Work out the finished part from the listing and answer in its coordinate system (mm). A direction names the side the tool comes from. Round coordinates to 2 decimals unless told otherwise and drop trailing zeros. Order: outer loops, then holes, each group sorted by start corner. A loop starts at its lowest first (then second) coordinate and runs counter-clockwise, first axis right, second up. Notation, with made-up numbers: (64, 85.25) - (109, 85.25) arc R22 ccw to (109, 120.25) - close; hole circle Ø6 at (74.25, 4). An arc over 180 degrees is marked (long way). Use CSV: the item, a comma, the result in double quotes.
from build123d import *

# Parameters (mm, degrees)
BOSS_EXTRUDE1_DEPTH          = 350
F_3_0_3_DIAMETER_SLOT1_D     = 3
F_3_0_3_DIAMETER_HOLE2_D     = 3
F_3_0_3_DIAMETER_HOLE2_DEPTH = 4


with BuildPart() as part:
    # Sketch1 → Boss-Extrude1 (new body)
    with BuildSketch(Plane(origin=(0, 0, 0), x_dir=(1, 0, 0), z_dir=(0, 1, 0))):
        Polygon((0, 0), (0, 10), (2, 10), (2, 2), (20, 2), (20, 0), align=None)
    extrude(amount=BOSS_EXTRUDE1_DEPTH)

    # Ø3.0 (3) Diameter Slot1 (through all)
    with Locations(Plane.XY):
        with Locations((14.838501141, 25.910104069), (14.838501141, 323.866264903)):
            Hole(F_3_0_3_DIAMETER_SLOT1_D / 2)

    # Ø3.0 (3) Diameter Hole2
    with Locations(Plane(origin=(0, 128.861996081, -176.67995168), x_dir=(0, 1, 0), z_dir=(-1, 0, 0))):
        with Locations((-122.861996081, -170.67995168), (-108.861996081, -170.67995168), (215.138003919, -170.67995168), (201.138003919, -170.67995168)):
            Hole(F_3_0_3_DIAMETER_HOLE2_D / 2, depth=F_3_0_3_DIAMETER_HOLE2_DEPTH)


solid = part.part
(1) For faces 1 (the flat face through (2, 173, -6)), 2 (the flat face through (10, 173, 0)), determine the directions among +Z, -Z, +X, -X, +Y, -Y from which every point of the face is accessible in a straight line to the end or side of a thin tool.
Findings below:
face 1,"-Z, +X, +Y, -Y"
face 2,"+Z, +X, -X, +Y, -Y"
(2) Find the intervals of material crossed by L1, parallel to Z at x = 0.8, y = 20; L2, parallel to Y at x = 1.15, z = -6; L3, parallel to X at y = 302, z = -6.75, in increasing order. Write a range as from..to.
Findings below:
L1,"z = -10..-7.5, -4.5..0"
L2,"y = 0..4.5, 7.5..18.5, 21.5..328.5, 331.5..342.5, 345.5..350"
L3,"x = 0..2"
(3) Find section A-A (z = -6). Determine the outline of the cut face in (x, y), and give its area (3 significant figures).
Findings below:
outline,"(0, 0) - (2, 0) - (2, 4.5) - (0, 4.5) - close; (0, 7.5) - (2, 7.5) - (2, 18.5) - (0, 18.5) - close; (0, 21.5) - (2, 21.5) - (2, 328.5) - (0, 328.5) - close; (0, 331.5) - (2, 331.5) - (2, 342.5) - (0, 342.5) - close; (0, 345.5) - (2, 345.5) - (2, 350) - (0, 350) - close"
area,"676 mm²"
(4) Each of these flat-tipped pins is pushed along its axis until it touches: pin 1 (2.5 mm diameter, centred on x = 14.84, y = 323.87, fed in from +Z); pin 2 (6 mm diameter, centred on x = 12, y = 307, fed in from -Z); pin 3 (3.5 mm diameter, centred on y = 344, z = -6, fed in from +X). Where does it stop, or does it pass through?
Findings below:
pin 1,"passes through"
pin 2,"stops at z = -2"
pin 3,"stops at x = 2"
